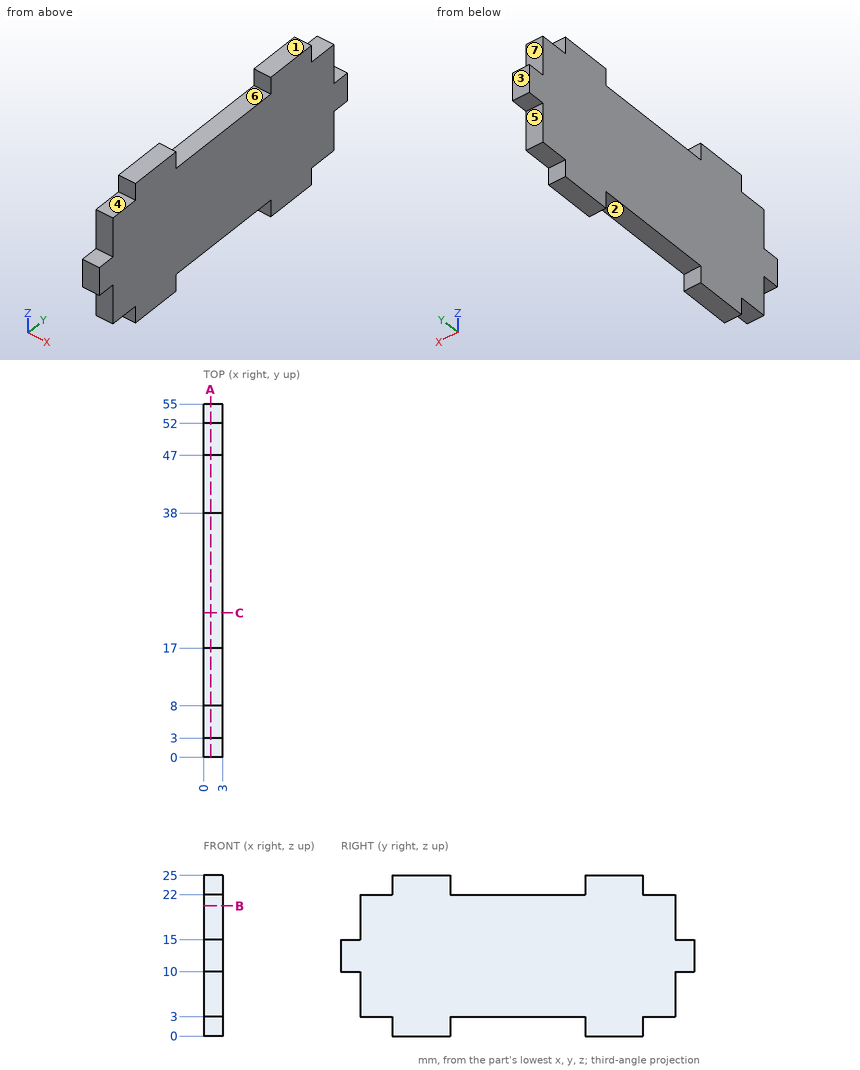
For this review, use the dimensioned drawing (mm, ordinates from the lowest corner) and the shaded views. A direction names the side the tool comes from. Coordinates: 2 decimals unless noted, no trailing zeros. Write each loop counter-clockwise with the first axis right and the second up, starting at its lowest first coordinate (ties: lowest second). Pieces come first, ordered by that corner, then holes. Notation, with made-up numbers: (10, 47.5) - (29, 47.5) arc R19 cw to (29, 63.5) - close; hole circle Ø7 at (46, -35). An arc over 180 degrees is marked (long way). Answer in a Markdown table with one row per item. Add a question column.
Q1. Consider section C-C on y = 22.5. Give the boundary of the cut face in (x, z).
Q2. Clearance check with flat-ended pins moving along their axes: pin 1 (1.5 mm diameter, centred on x = 1, z = 18, fed in from +Y); pin 2 (1.5 mm diameter, centred on x = 2, z = 1.5, fed in from -Y); pin 3 (6 mm diameter, centred on y = 14, z = 10, fed in from -X); pin 4 (1.5 mm diameter, centred on x = 1.5, z = 2, fed in from +Y). State where each tip first meets the part, or that it passes through.
Q3. For the marked faces 4, 5, 6 and 7, list the 3-axis set-ups (+Z, -Z, +X, -X, +Y, -Y) from which the entire face can be reached by the end or side of a thin tool; tool diameter is ignored.
Q4. Consider section A-A on x = 1.1. Give the boundary of the cut face in (y, z), then the cut area to 3 significant figures.
Q5. Consider section B-B on z = 20.25. Give the boundary of the cut face in (x, y), then the cut area to 3 significant figures.
Q6. To check wall thickness, follow line 1 along Y through (x, z) = (2.3, 1); line 2 along Y through (x, z) = (2, 6); line 3 along Z through (x, y) = (1.95, 50). State the ranges of each line that lie inside material, in increasing order. Write a range as from..to.
Q7. Draft analysis for pull direction Y (two halves, no side actions). For the marked faces 1, 2 and 3, state which applies: +Y half, -Y half, draft (parallel to the pull), parting line (faces both ways), or undercut.
Answers below:
| question | item | result |
|---|---|---|
| 1 | outline | (0, 3) - (3, 3) - (3, 22) - (0, 22) - close |
| 2 | pin 1 | y = 52 |
| 2 | pin 2 | y = 8 |
| 2 | pin 3 | x = 0 |
| 2 | pin 4 | y = 47 |
| 3 | face 4 | +Z, +X, -X, -Y |
| 3 | face 5 | -Z, +X, -X, +Y |
| 3 | face 6 | +Z, +X, -X |
| 3 | face 7 | +Z, +X, -X, +Y |
| 4 | outline | (0, 10) - (3, 10) - (3, 3) - (8, 3) - (8, 0) - (17, 0) - (17, 3) - (38, 3) - (38, 0) - (47, 0) - (47, 3) - (52, 3) - (52, 10) - (55, 10) - (55, 15) - (52, 15) - (52, 22) - (47, 22) - (47, 25) - (38, 25) - (38, 22) - (17, 22) - (17, 25) - (8, 25) - (8, 22) - (3, 22) - (3, 15) - (0, 15) - close |
| 4 | area | 1,070 mm² |
| 5 | outline | (0, 3) - (3, 3) - (3, 52) - (0, 52) - close |
| 5 | area | 147 mm² |
| 6 | line 1 | 8..17, 38..47 |
| 6 | line 2 | 3..52 |
| 6 | line 3 | 3..22 |
| 7 | face 1 | draft |
| 7 | face 2 | undercut |
| 7 | face 3 | +Y half |
